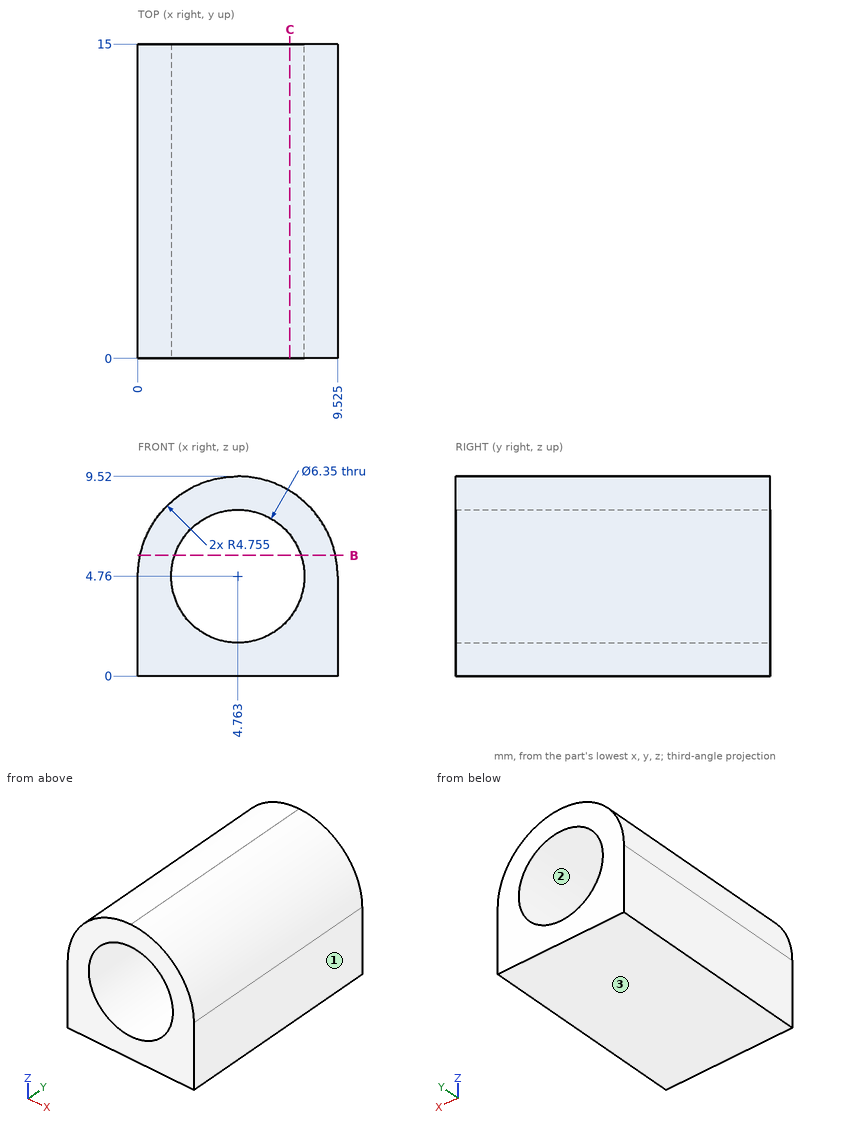
For this review, use the dimensioned drawing (mm, ordinates from the lowest corner) and the shaded views. Give positions to 0.01 mm unless a question says otherwise; leave off trailing zeros. Write each loop counter-clockwise with the first axis right and the second up, starting at its lowest first coordinate (ties: lowest second). Pieces come first, ordered by that corner, then holes. Notation, with made-up numbers: M 34,79.25 L 91,79.25 A29 cw 91,108.25 Z; hole C 4.25,27 d6. An arc over 180 degrees is marked long. Answer as a JSON object with one key per item and string values. Group by question number.
Item 1: For pin 1 Ø5 at (x, z) = (4.76, 4.76) entering from -Y; pin 2 Ø1 at (x, y) = (7, 6) entering from +Z (1 decimal), all flat-tipped, find the tip position at first contact; note any pin that passes through.
Item 2: Consider section B-B on z = 5.75. Write out the cut boundary in (x, y) (1 decimal).
Item 3: Consider section C-C on x = 7.25. Write out the cut boundary in (y, z).
Item 4: For probe 1 along X at (y, z) = (5.75, 4) (1 decimal); probe 2 along X at (y, z) = (5, 5) (1 decimal); probe 3 along Z at (x, y) = (6.25, 8.75) (1 decimal), list the stretches that pass through material, from the lowest coordinate up. Write a range as [from, to].
Item 5: Draft analysis for pull direction X (two halves, no side actions). For the marked faces 1, 2 and 3, state which applies: +X half, -X half, draft (parallel to the pull), parting line (faces both ways), or undercut.
Check result:
{
 "1": {"pin 1": "passes through", "pin 2": "stops at z = 9.2"},
 "2": {"outline": "M 0.1,0 L 1.7,0 L 1.7,15 L 0.1,15 Z; M 7.8,0 L 9.4,0 L 9.4,15 L 7.8,15 Z"},
 "3": {"outline": "M 0,0 L 15,0 L 15,2.79 L 0,2.79 Z; M 0,6.73 L 15,6.73 L 15,8.82 L 0,8.82 Z"},
 "4": {"probe 1": "x = [0, 1.7], [7.8, 9.5]", "probe 2": "x = [0, 1.6], [7.9, 9.5]", "probe 3": "z = [0, 2], [7.6, 9.3]"},
 "5": {"face 1": "+X half", "face 2": "undercut", "face 3": "draft"}
}
